from build123d import *

# Parameters (mm, degrees)
ESQUISSE1_R      = 7.25
EXTRUSION1_DEPTH = 0.85


with BuildPart() as part:
    # Esquisse1 → Extrusion1 (new body, symmetric)
    with BuildSketch(Plane.XY):
        Circle(ESQUISSE1_R)
        with BuildLine():
            Line((-3, 2.645751311), (-3, -2.645751311))
            ThreePointArc((-3, -2.645751311), (0, -4), (3, -2.645751311))
            Line((3, -2.645751311), (3, 2.645751311))
            ThreePointArc((3, 2.645751311), (0, 4), (-3, 2.645751311))
        make_face(mode=Mode.SUBTRACT)
    extrude(amount=EXTRUSION1_DEPTH, both=True)


solid = part.part
Here's how the part is built. I have some questions about the finished solid (model axes, mm). A direction names the side the tool comes from. Round coordinates to 2 decimals unless told otherwise and drop trailing zeros. Write each loop counter-clockwise with the first axis right and the second up, starting at its lowest first coordinate (ties: lowest second). Pieces come first, ordered by that corner, then holes.
1. If we mould it in two halves opening along Y, with no side actions, what happens to faces 3 (the cylindrical face through (3.35, -6.43, 0.01)), 4 (the flat face through (-3.3, 0.1, -0.85)), 5 (the cylindrical face through (0, -4, 0))? For each: released by +Y, released by -Y, zero draft, split by the parting line, or undercut.
2. Suppose I cut it at D-D (x = 3.5). List the corners of the cut face in (y, z) for me.
3. I need wall thicknesses on L1, parallel to Y at x = -1.25, z = -0.4; L2, parallel to Y at x = -1, z = 0.35; L3, parallel to X at y = 2, z = 0.05. Which ranges of each line are inside material? Lowest first, please.
4. Suppose I cut it at C-C (z = 0.3). List the corners of the cut face in (x, y) for me.
5. Suppose I cut it at A-A (x = 0). List the corners of the cut face in (y, z) for me, and give its area (4 significant figures).
6. For faces 1 (the flat face through (-3, 0, 0)), 2 (the flat face through (-3.3, 0.1, 0.85)), which set-ups out of +Z, -Z, +X, -X, +Y, -Y let a thin tool reach every point of the face, with its end or its side?
7. Suppose I cut it at B-B (y = 0). List the corners of the cut face in (x, z) for me, and give its area (4 significant figures).
8. Will this pin go through, and if not, where does the flat tip stop? pin 1 Ø1 at (x, z) = (1, 0.5) entering from -Y.
Answer sheet:
1. face 3: split by the parting line
1. face 4: zero draft
1. face 5: undercut
2. outline: (-6.35, -0.85) - (6.35, -0.85) - (6.35, 0.85) - (-6.35, 0.85) - close
3. L1: y = -7.14 to -3.8, 3.8 to 7.14
3. L2: y = -7.18 to -3.87, 3.87 to 7.18
3. L3: x = -6.97 to -3, 3 to 6.97
4. outline: circle Ø14.5 at (0, 0); hole (-3, -2.65) arc R4 ccw to (3, -2.65) - (3, 2.65) arc R4 ccw to (-3, 2.65) - close
5. outline: (-7.25, -0.85) - (-4, -0.85) - (-4, 0.85) - (-7.25, 0.85) - close; (4, -0.85) - (7.25, -0.85) - (7.25, 0.85) - (4, 0.85) - close
5. area: 11.05 mm2
6. face 1: +Z, -Z
6. face 2: +Z, +X, -X, +Y, -Y
7. outline: (-7.25, -0.85) - (-3, -0.85) - (-3, 0.85) - (-7.25, 0.85) - close; (3, -0.85) - (7.25, -0.85) - (7.25, 0.85) - (3, 0.85) - close
7. area: 14.45 mm2
8. pin 1: stops at y = -7.23
